The listing builds one solid part. Answer for the finished solid, in the listing's coordinates (mm). A direction names the side the tool comes from. Round coordinates to 2 decimals unless told otherwise and drop trailing zeros. Write each loop counter-clockwise with the first axis right and the second up, starting at its lowest first coordinate (ties: lowest second). Pieces come first, ordered by that corner, then holes. Notation, with made-up numbers: M 89.25,-29.5 L 119.25,-29.5 A23 cw 119.25,-2.5 Z; hole C -15,40 d11. An arc over 180 degrees is marked long. Write each question's results on one line, items separated by ' | '.
from build123d import *

# Parameters (mm, degrees)
SKETCH2_W           = 42.3
SKETCH2_H           = 42.3
BOSS_EXTRUDE2_DEPTH = 39.8
SKETCH4_R           = 11
BOSS_EXTRUDE3_DEPTH = 2.032
SKETCH6_R           = 1.5
CUT_EXTRUDE1_DEPTH  = 2
SKETCH7_W           = 16
SKETCH7_H           = 11
BOSS_EXTRUDE4_DEPTH = 7
SKETCH9_R           = 2.5
BOSS_EXTRUDE5_DEPTH = 15
BOSS_EXTRUDE7_START = -11
SKETCH11_R          = 8
SKETCH11_R_2        = 2.5
BOSS_EXTRUDE7_DEPTH = 11
SKETCH13_R          = 2.5
BOSS_EXTRUDE8_DEPTH = 0.8


with BuildPart() as part:
    # Sketch2 → Boss-Extrude2 (new body)
    with BuildSketch(Plane(origin=(0, 0, 0), x_dir=(1, 0, 0), z_dir=(0, 1, 0))):
        Rectangle(SKETCH2_W, SKETCH2_H)
    extrude(amount=BOSS_EXTRUDE2_DEPTH)

    # Sketch4 → Boss-Extrude3 (add)
    with BuildSketch(Plane.XZ):
        with Locations(Location((0, 0, 0), (0, 0, 270))):
            Circle(SKETCH4_R)
    extrude(amount=BOSS_EXTRUDE3_DEPTH)

    # Sketch6 → Cut-Extrude1 (cut)
    with BuildSketch(Plane.XZ):
        with Locations(Location((15.5, 15.5, 0), (0, 0, 270))):
            Circle(SKETCH6_R)
        with Locations(Location((-15.5, 15.5, 0), (0, 0, 270))):
            Circle(SKETCH6_R)
        with Locations(Location((-15.5, -15.5, 0), (0, 0, 270))):
            Circle(SKETCH6_R)
        with Locations(Location((15.5, -15.5, 0), (0, 0, 270))):
            Circle(SKETCH6_R)
    extrude(amount=-CUT_EXTRUDE1_DEPTH, mode=Mode.SUBTRACT)

    # Sketch7 → Boss-Extrude4 (add)
    with BuildSketch(Plane.XY.offset(21.15)):
        with Locations((0, 34.3)):
            Rectangle(SKETCH7_W, SKETCH7_H)
    extrude(amount=BOSS_EXTRUDE4_DEPTH)

    # Sketch9 → Boss-Extrude5 (add)
    with BuildSketch(Plane.XZ.offset(2.032)):
        with Locations(Location((0, 0, 0), (0, 0, 270))):
            Circle(SKETCH9_R)
    extrude(amount=BOSS_EXTRUDE5_DEPTH)

    # Sketch11 → Boss-Extrude7 (add)
    with BuildSketch(Plane.XZ.offset(17.032).offset(BOSS_EXTRUDE7_START)):
        with Locations(Location((0, 0, 0), (0, 0, 270))):
            Circle(SKETCH11_R)
        with Locations(Location((0, 0, 0), (0, 0, 270))):
            Circle(SKETCH11_R_2, mode=Mode.SUBTRACT)
    extrude(amount=BOSS_EXTRUDE7_DEPTH)

    # Sketch13 → Boss-Extrude8 (add)
    with BuildSketch(Plane.XZ.offset(17.032)):
        with Locations(Location((0, 0, 0), (0, 0, 270))):
            Circle(SKETCH13_R)
    extrude(amount=BOSS_EXTRUDE8_DEPTH)


solid = part.part
1) A tool of negligible diameter and unlimited length cuts with its end or side. For faces 1 (the face through (2, -6.032, -2)), 2 (the face through (-15, 2, -15)), 3 (the face through (-8, 34, 25)), from which of +Z, -Z, +X, -X, +Y, -Y can it reach the whole face along a straight path? Write none if from no direction.
Return value:
face 1: none | face 2: -Y | face 3: +Z, -X, +Y, -Y
2) Each of these flat-tipped pins is pushed along its axis until it touches: pin 1 (1.5 mm diameter, centred on x = 15.5, z = -15, fed in from -Y); pin 2 (5.5 mm diameter, centred on y = 32, z = 23, fed in from +X); pin 3 (3.5 mm diameter, centred on x = -15.5, z = -15.5, fed in from -Y); pin 4 (4 mm diameter, centred on x = -11.5, y = 10, fed in from +Z). Where does it stop, or does it pass through?
Return value:
pin 1: y = 2 | pin 2: x = 21.15 | pin 3: y = 0 | pin 4: z = 21.15
3) Section B-B (z = 15.5) is taken. Determine the outline of the cut face in (x, y), then the cut area to 3 significant figures.
Return value:
outline: M -21.15,0 L -17,0 L -17,2 L -14,2 L -14,0 L 14,0 L 14,2 L 17,2 L 17,0 L 21.15,0 L 21.15,39.8 L -21.15,39.8 Z | area: 1,670 mm²
4) Find the intervals of material crossed by line 1 (X direction, y = 1.4, z = -15.5); line 2 (Y direction, x = -1, z = 9); line 3 (Y direction, x = 17, z = 3.5), in increasing order.
Return value:
line 1: -21.15 to -17, -14 to 14, 17 to 21.15 | line 2: -2.03 to 39.8 | line 3: 0 to 39.8
5) Section C-C (y = 30.5) is taken. Determine the outline of the cut face in (x, z).
Return value:
outline: M -21.15,-21.15 L 21.15,-21.15 L 21.15,21.15 L 8,21.15 L 8,28.15 L -8,28.15 L -8,21.15 L -21.15,21.15 Z
6) Section D-D (x = -4.5) is taken. Determine the outline of the cut face in (y, z), then the cut area to 3 significant figures.
Return value:
outline: M -17.03,-6.61 L -6.03,-6.61 L -6.03,6.61 L -17.03,6.61 Z; M -2.03,-10.04 L 0,-10.04 L 0,-21.15 L 39.8,-21.15 L 39.8,28.15 L 28.8,28.15 L 28.8,21.15 L 0,21.15 L 0,10.04 L -2.03,10.04 Z | area: 1,950 mm²
7) The mould has two halves that part along Y. Classify faces 4 (the face through (0, 39.8, 3)), 5 (the face through (0, -2.032, 3)), 6 (the face through (-15, 2, 16)): +Y half, -Y half, draft (parallel to the pull), parting line (faces both ways), or undercut.
Return value:
face 4: +Y half | face 5: undercut | face 6: -Y half
8) Section A-A (x = 0) is taken. Determine the outline of the cut face in (y, z).
Return value:
outline: M -17.83,-2.5 L -17.03,-2.5 L -17.03,-8 L -6.03,-8 L -6.03,-2.5 L -2.03,-2.5 L -2.03,-11 L 0,-11 L 0,-21.15 L 39.8,-21.15 L 39.8,28.15 L 28.8,28.15 L 28.8,21.15 L 0,21.15 L 0,11 L -2.03,11 L -2.03,2.5 L -6.03,2.5 L -6.03,8 L -17.03,8 L -17.03,2.5 L -17.83,2.5 Z
